Check sheet for the modelled part. Datum: model origin and axes. Units: mm. Face numbers are marked on the shaded views. A direction names the side the tool comes from. Coordinates: 2 decimals unless noted, no trailing zeros. Loops run counter-clockwise (first coordinate to the right, second up) from the corner with the lowest first, then second, coordinate; pieces in that order, holes last.
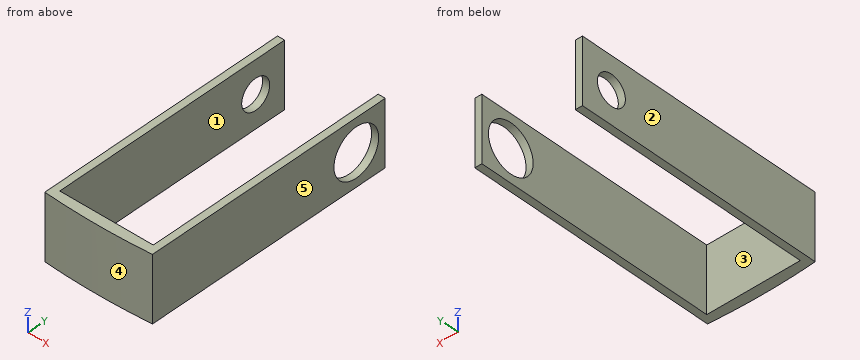
```python
from build123d import *

# Parameters (mm, degrees)
BOSS_EXTRUDE1_DEPTH       = 5.842
F_6_32_TAPPED_HOLE1_D     = 2.7051
F_6_32_TAPPED_HOLE1_DEPTH = 0.635
CUT_EXTRUDE1_REACH        = 11.652
SKETCH6_R                 = 2.159
BOSS_EXTRUDE2_DEPTH       = 5.842


with BuildPart() as part:
    # Sketch1 → Boss-Extrude1 (new body)
    with BuildSketch(Plane.XY):
        Polygon((-3.353873239, 20.18718662), (-3.353873239, -2.29181338), (6.298126761, -2.29181338), (6.298126761, 20.18718662), (5.663126761, 20.18718662), (5.663126761, -1.52981338), (-2.718873239, -1.52981338), (-2.718873239, 20.18718662), align=None)
    extrude(amount=BOSS_EXTRUDE1_DEPTH)

    # #6-32 Tapped Hole1
    with Locations(Plane.ZY.offset(3.353873239)):
        with Locations((2.921, 17.39318662)):
            Hole(F_6_32_TAPPED_HOLE1_D / 2, depth=F_6_32_TAPPED_HOLE1_DEPTH)

    # Sketch6 → Cut-Extrude1 (cut, up to next)
    with BuildSketch(Plane(origin=(6.298126761, 0, 0), x_dir=(0, 0, -1), z_dir=(1, 0, 0)), mode=Mode.PRIVATE) as cut_extrude1_sk1:
        with Locations((-2.921, 17.39318662)):
            Circle(SKETCH6_R)
    cut_extrude1_tool1 = extrude(cut_extrude1_sk1.sketch, amount=-CUT_EXTRUDE1_REACH, mode=Mode.PRIVATE) & part.part
    add(cut_extrude1_tool1.solids().sort_by_distance((6.298127, 17.393187, 2.921))[0], mode=Mode.SUBTRACT)

    # Sketch15 → Boss-Extrude2 (add, through all)
    with BuildSketch(Plane.XY):
        with BuildLine():
            Line((6.298126761, -2.29181338), (-3.353873239, -2.29181338))
            ThreePointArc((-3.353873239, -2.29181338), (1.472126761, -2.477704159), (6.298126761, -2.29181338))
        make_face()
    extrude(amount=BOSS_EXTRUDE2_DEPTH)


solid = part.part
```
1) Depth check by flat-ended pin: pin 1 (3 mm diameter, centred on x = -1.5, z = 4.5, fed in from -Y); pin 2 (1.8 mm diameter, centred on x = 2, z = 2, fed in from +Y). Enter the tip coordinate at first touch or a pass-through.
Answer sheet:
pin 1: stops at y = -2.46
pin 2: stops at y = -1.53
2) Set-up check for the marked faces 1 and 2: record each of +Z, -Z, +X, -X, +Y, -Y from which the full face is reachable in a straight line by a thin tool's end or side.
Answer sheet:
face 1: +Z, -Z, +Y
face 2: +Z, -Z, -X, +Y, -Y
3) Section check C-C on z = 2.5. Enter the section's corners in (x, y).
Answer sheet:
outline: (-3.35, -2.29) arc R62.74 ccw to (6.3, -2.29) - (6.3, 15.28) - (5.66, 15.28) - (5.66, -1.53) - (-2.72, -1.53) - (-2.72, 16.11) - (-3.35, 16.11) - close; (-3.35, 18.68) - (-2.72, 18.68) - (-2.72, 20.19) - (-3.35, 20.19) - close; (5.66, 19.51) - (6.3, 19.51) - (6.3, 20.19) - (5.66, 20.19) - close
4) Section check A-A on y = 12.25. Enter the section's corners in (x, z).
Answer sheet:
outline: (-3.35, 0) - (-2.72, 0) - (-2.72, 5.84) - (-3.35, 5.84) - close; (5.66, 0) - (6.3, 0) - (6.3, 5.84) - (5.66, 5.84) - close
5) Section check D-D on y = 18. Enter the section's corners in (x, z), plus the area to 3 significant figures.
Answer sheet:
outline: (-3.35, 0) - (-2.72, 0) - (-2.72, 1.71) - (-3.35, 1.71) - close; (-3.35, 4.13) - (-2.72, 4.13) - (-2.72, 5.84) - (-3.35, 5.84) - close; (5.66, 0) - (6.3, 0) - (6.3, 0.85) - (5.66, 0.85) - close; (5.66, 4.99) - (6.3, 4.99) - (6.3, 5.84) - (5.66, 5.84) - close
area: 3.25 mm2
6) Scan lines: line 1 (X direction, y = 9, z = 3.7); line 2 (Y direction, x = 1, z = 4.1); line 3 (Y direction, x = 5.75, z = 3.9). Record each from-to range of solid material in increasing order.
Answer sheet:
line 1: x = -3.35 to -2.72, 5.66 to 6.3
line 2: y = -2.48 to -1.53
line 3: y = -2.33 to 15.47, 19.32 to 20.19
7) Mould release check, pull along X, two halves, no side actions. Record for the marked faces 3, 4 and 5: +X half, -X half, draft (parallel to the pull), parting line (faces both ways), or undercut.
Answer sheet:
face 3: undercut
face 4: parting line
face 5: +X half
8) Section check B-B on z = 1. Enter the section's corners in (x, y), plus the area to 3 significant figures.
Answer sheet:
outline: (-3.35, -2.29) arc R62.74 ccw to (6.3, -2.29) - (6.3, 16.41) - (5.66, 16.41) - (5.66, -1.53) - (-2.72, -1.53) - (-2.72, 20.19) - (-3.35, 20.19) - close; (5.66, 18.38) - (6.3, 18.38) - (6.3, 20.19) - (5.66, 20.19) - close
area: 34.9 mm2
